Part model, mm, in its own coordinate system. Face numbers are marked on the shaded views. A direction names the side the tool comes from. Coordinates: 2 decimals unless noted, no trailing zeros. Write each loop counter-clockwise with the first axis right and the second up, starting at its lowest first coordinate (ties: lowest second). Pieces come first, ordered by that corner, then holes. Notation, with made-up numbers: (25, 16.5) -> (72, 16.5) arc R7 cw to (72, 20.5) -> close; hole circle Ø9 at (67, 75). An arc over 180 degrees is marked (long way). Write item = value, one per line. Start each with the question number.
Q1. Pin check, flat tip, straight feed: P1, Ø3, axis at x = 6.5, y = -8, coming from the +Z side. Stop position of the tip, or through.
Q2. Probe line 1 (Z direction, x = 4, y = -9); line 2 (X direction, y = -28, z = 16); line 3 (Z direction, x = -0.5, y = -27). List the from-to ranges inside material, lowest first.
Q3. Tool access for the marked faces 1 and 2: list every direction of +Z, -Z, +X, -X, +Y, -Y with a clear straight run to the whole face (end or side of a thin tool).
Q4. Band-saw the part on B-B, the plane z = 6.5. List the corners of the cut face in (x, y), plus the area to 3 significant figures.
Q5. Band-saw the part on C-C, the plane x = 3. List the corners of the cut face in (y, z).
Q6. Band-saw the part on A-A, the plane y = -25.5. List the corners of the cut face in (x, z), plus the area to 3 significant figures.
from build123d import *

# Parameters (mm, degrees)
F1_DEPTH = 30
F2_SIZE  = 1


# Not quite as in the source:
# - a feature names something its author has since deleted; it is built from what else it names


with BuildPart() as f1:
    # F0 (on Front) → F1 (new body)
    with BuildSketch(Plane.XZ):
        Polygon((19, 0), (0, 0), (0, 24), (-19, 24), (-19, -24), (19, -24), align=None)
    extrude(amount=F1_DEPTH)

    # F2
    f2_edges = [f1.edges().sort_by_distance(p)[0] for p in [
        (9.5, -30, 0),
        (0, -30, 12),
        (-9.5, -30, 24),
        (-19, -30, 0),
        (0, -30, -24),
        (19, -30, -12),
        (9.5, 0, 0),
        (0, 0, 12),
        (-9.5, 0, 24),
        (-19, 0, 0),
        (0, 0, -24),
        (19, 0, -12),
        (0, -15, 24),
        (-19, -15, 24),
        (-19, -15, -24),
        (19, -15, -24),
        (19, -15, 0),
    ]]
    chamfer(f2_edges, length=F2_SIZE)


solid = f1.part
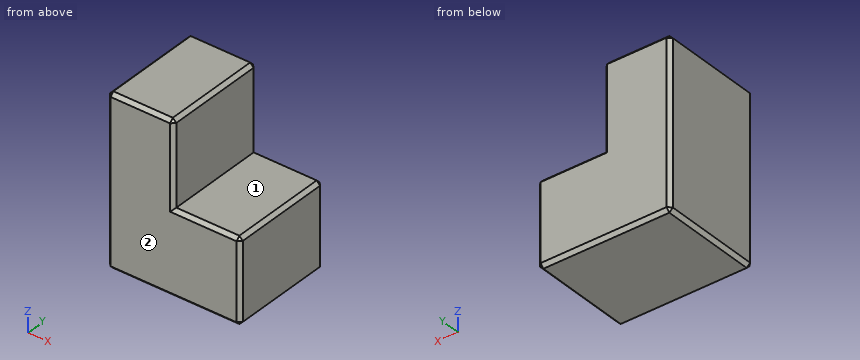
Ans:
q1.P1 = 0
q2.line_1 = -24 to 0
q2.line_2 = -19 to 0
q2.line_3 = -24 to 23.5
q3.face_1 = +Z, +X, +Y, -Y
q3.face_2 = +Z, -Z, +X, -X, -Y
q4.outline = (-19, -29) -> (-18, -30) -> (-1, -30) -> (0, -29) -> (0, -1) -> (-1, 0) -> (-18, 0) -> (-19, -1) -> close
q4.area = 568 mm2
q5.outline = (-30, -23) -> (-29, -24) -> (-1, -24) -> (0, -23) -> (0, -1) -> (-1, 0) -> (-29, 0) -> (-30, -1) -> close
q6.outline = (-19, -23) -> (-18, -24) -> (18, -24) -> (19, -23) -> (19, -1) -> (18, 0) -> (0, 0) -> (0, 23) -> (-1, 24) -> (-18, 24) -> (-19, 23) -> close
q6.area = 1,370 mm2
